Source: CAD feature listing. Evaluate the final solid. Frame: model axes, mm. Give positions to 0.01 mm unless a question says otherwise; leave off trailing zeros. Write each loop counter-clockwise with the first axis right and the second up, starting at its lowest first coordinate (ties: lowest second). Pieces come first, ordered by that corner, then holes.
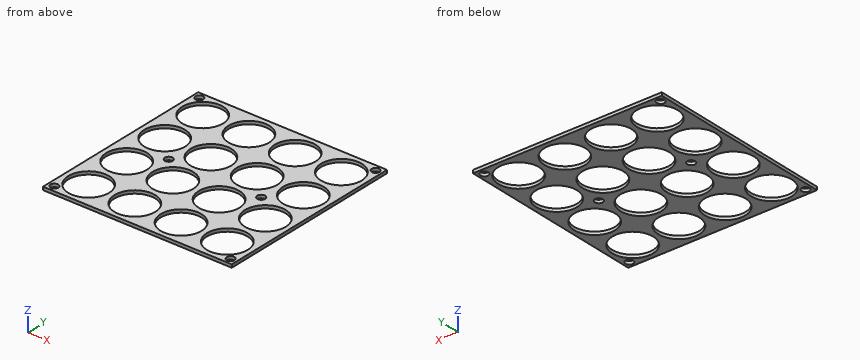
```python
from build123d import *

# Parameters (mm, degrees)
F0_W     = 122.5
F0_H     = 122.5
F0_R     = 2.55
F0_R_2   = 13.25
F1_DEPTH = 2


with BuildPart() as f1:
    # F0 (on Top) → F1 (new body)
    with BuildSketch(Plane.XY):
        Rectangle(F0_W, F0_H)
        with Locations((-57.2, -57.2)):
            Circle(F0_R, mode=Mode.SUBTRACT)
        with Locations((-45, -45)):
            Circle(F0_R_2, mode=Mode.SUBTRACT)
        with Locations((-15, -45)):
            Circle(F0_R_2, mode=Mode.SUBTRACT)
        with Locations((-45, -15)):
            Circle(F0_R_2, mode=Mode.SUBTRACT)
        with Locations((-15, -15)):
            Circle(F0_R_2, mode=Mode.SUBTRACT)
        with Locations((15, -45)):
            Circle(F0_R_2, mode=Mode.SUBTRACT)
        with Locations((57.2, -57.2)):
            Circle(F0_R, mode=Mode.SUBTRACT)
        with Locations((45, -45)):
            Circle(F0_R_2, mode=Mode.SUBTRACT)
        with Locations((15, -15)):
            Circle(F0_R_2, mode=Mode.SUBTRACT)
        with Locations((45, -15)):
            Circle(F0_R_2, mode=Mode.SUBTRACT)
        with Locations((-45, 15)):
            Circle(F0_R_2, mode=Mode.SUBTRACT)
        with Locations((-30, 0)):
            Circle(F0_R, mode=Mode.SUBTRACT)
        with Locations((-15, 15)):
            Circle(F0_R_2, mode=Mode.SUBTRACT)
        with Locations((-45, 45)):
            Circle(F0_R_2, mode=Mode.SUBTRACT)
        with Locations((-57.2, 57.2)):
            Circle(F0_R, mode=Mode.SUBTRACT)
        with Locations((-15, 45)):
            Circle(F0_R_2, mode=Mode.SUBTRACT)
        with Locations((15, 15)):
            Circle(F0_R_2, mode=Mode.SUBTRACT)
        with Locations((30, 0)):
            Circle(F0_R, mode=Mode.SUBTRACT)
        with Locations((45, 15)):
            Circle(F0_R_2, mode=Mode.SUBTRACT)
        with Locations((15, 45)):
            Circle(F0_R_2, mode=Mode.SUBTRACT)
        with Locations((45, 45)):
            Circle(F0_R_2, mode=Mode.SUBTRACT)
        with Locations((57.2, 57.2)):
            Circle(F0_R, mode=Mode.SUBTRACT)
    extrude(amount=F1_DEPTH)


solid = f1.part
```
1. Section query B-B (y = 24.5). Return loops of the section in (x, z).
2. Section query C-C (z = 0.4). Give the number of separate pieces and of enclosed holes in the cut face, plus the area to 3 significant figures.
3. Section query A-A (x = -45). Return loops of the section in (y, z), plus the area to 3 significant figures.
4. Pin query (flat end, axial travel): P1, Ø16, axis at x = 15, y = -15, coming from the -Z side. Return the tip coordinate at first contact, or that it passes through.
5. Line query: probe 1 along Y at (x, z) = (-15, 0.5); probe 2 along Y at (x, z) = (-22.5, 1.45); probe 3 along X at (y, z) = (5, 1.6). Output: solid intervals per line, ascending.
The answers:
1. outline: (-61.25, 0) - (-54.24, 0) - (-54.24, 2) - (-61.25, 2) - close; (-35.76, 0) - (-24.24, 0) - (-24.24, 2) - (-35.76, 2) - close; (-5.76, 0) - (5.76, 0) - (5.76, 2) - (-5.76, 2) - close; (24.24, 0) - (35.76, 0) - (35.76, 2) - (24.24, 2) - close; (54.24, 0) - (61.25, 0) - (61.25, 2) - (54.24, 2) - close
2. separate pieces: 1
2. enclosed holes: 22
2. area: 6,060 mm2
3. outline: (-61.25, 0) - (-58.25, 0) - (-58.25, 2) - (-61.25, 2) - close; (-31.75, 0) - (-28.25, 0) - (-28.25, 2) - (-31.75, 2) - close; (-1.75, 0) - (1.75, 0) - (1.75, 2) - (-1.75, 2) - close; (28.25, 0) - (31.75, 0) - (31.75, 2) - (28.25, 2) - close; (58.25, 0) - (61.25, 0) - (61.25, 2) - (58.25, 2) - close
3. area: 33.0 mm2
4. P1: passes through
5. probe 1: y = -61.25 to -58.25, -31.75 to -28.25, -1.75 to 1.75, 28.25 to 31.75, 58.25 to 61.25
5. probe 2: y = -61.25 to -55.92, -34.08 to -25.92, -4.08 to 4.08, 25.92 to 34.08, 55.92 to 61.25
5. probe 3: x = -61.25 to -53.69, -36.31 to -23.69, -6.31 to 6.31, 23.69 to 36.31, 53.69 to 61.25
